Geometry check sheet. Reference: the model listing, model coordinates, mm. A direction names the side the tool comes from. Round coordinates to 2 decimals unless told otherwise and drop trailing zeros. Order: outer loops, then holes, each group sorted by start corner. A loop starts at its lowest first (then second) coordinate and runs counter-clockwise, first axis right, second up.
Autodesk Inventor part; units mm, degrees
ref_plane "YZ Plane" through (0, 0, 0) normal (1, 0, 0) x (0, 1, 0)
ref_plane "XZ Plane" through (0, 0, 0) normal (0, 1, 0) x (-1, 0, 0)
ref_plane "XY Plane" through (0, 0, 0) normal (0, 0, 1) x (1, 0, 0)
sketch "Szkic8" plane through (0, 0, 0) normal (0, 1, 0) x (-1, 0, 0)
  circle A0 centre (0, 0) radius 38.05
  circle A1 centre (0, 0) radius 36.85
  dimension "d53" = 76.1
  dimension "d54" = 1.2
extrude "Wyciągnięcie proste2" add sketch "Szkic8" along normal mid plane 220
sketch "Szkic13" plane through (0, 0, 0) normal (0, 0, 1) x (1, 0, 0)
  circle A0 centre (0, 0) radius 12.5
  circle A1 centre (0, 0) radius 11.3
  dimension "d67" = 25
  dimension "d68" = 1.2
extrude "Wyciągnięcie proste6" add sketch "Szkic13" along normal blind 41
sketch "Szkic14" plane through (0, 0, 41) normal (0, 0, 1) x (1, 0, 0)
  circle A0 centre (0, 0) radius 11.3
extrude "Wyciągnięcie proste7" cut sketch "Szkic14" against normal blind 41
sketch "Szkic15" plane through (0, -110, 0) normal (0, -1, 0) x (1, 0, 0)
  circle A0 centre (0, 0) radius 36.85
extrude "Wyciągnięcie proste8" cut sketch "Szkic15" against normal blind 220
fillet "Zaokrąglenie3" radius 1.2 2 edges at (0, 12.5, 38.05) (0, -12.5, 38.05)
fillet "Zaokrąglenie4" radius 2.4 2 edges at (0.0022, -11.3, 36.85) (0, 11.3, 36.85)
equation "\"d53\" = OD"
equation "\"d54\" = THK"
equation "\"d55\" = L1"
equation "\"d67\" = OD2"
equation "\"d68\" = THK"
equation "\"d69\" = L2"
equation "\"d71\" = L2"
equation "\"d73\" = L1"
equation "\"d75\" = THK"
equation "\"d76\" = 2 * THK"
equation "\"SzerokośćGięciaPodcięcia\" = Grubość"
equation "\"RozmiarPodcięciaNarożnika\" = 4 * Grubość"
equation "\"PromieńPrzejścia\" = PromieńGięcia"
equation "\"Rozmiar_promienia_Jacobiego\" = PromieńGięcia"
equation "\"Wielk_odstępu\" = Grubość"
equation "\"d2\" = PromieńGięcia"
equation "\"d23\" = PromieńGięcia"
equation "\"OD\" = 76.1"
equation "\"THK\" = 1.2"
equation "\"L1\" = 220"
equation "\"L2\" = 41"
equation "\"OD2\" = 25"
properties part number "Trójnik red. krótki  Ø76,1 25 76,1 s=1,2 L=220" material "304"
(1) Draft check along Z on faces 3 (the cylindrical face through (-20.46, -1.54, -32.08)), 4 (the cylindrical face through (7.988, 1.54, -35.974)), 5 (the flat face through (-6, -10, 41)). Enter one of: released by +Z, released by -Z, zero draft, split by the parting line, or undercut.
Returned:
face 3: split by the parting line
face 4: undercut
face 5: released by +Z
(2) Material ranges on line 1 (Z direction, x = 0, y = -20); line 2 (X direction, y = 0, z = 39.65), recorded low to high.
Returned:
line 1: z = -38.05 to -36.85, 36.85 to 38.05
line 2: x = -12.5 to -11.3, 11.3 to 12.5
(3) Sectioned sample at D-D, the plane x = 0. Give the number of separate pieces and of enclosed holes in the cut face, and give its area (3 significant figures).
Returned:
separate pieces: 3
enclosed holes: 0
area: 506 mm2
(4) Sectioned sample at C-C, the plane y = 79.5. Record the cut outline in (x, z), and give its area (3 significant figures).
Returned:
outline: circle Ø76.1 at (0, 0); hole circle Ø73.7 at (0, 0)
area: 282 mm2
(5) Sectioned sample at A-A, the plane z = 0. Record the cut outline in (x, y), and give its area (3 significant figures).
Returned:
outline: (-38.05, -110) - (-36.85, -110) - (-36.85, 110) - (-38.05, 110) - close; (36.85, -110) - (38.05, -110) - (38.05, 110) - (36.85, 110) - close
area: 528 mm2
(6) Set-up check for faces 1 (the cylindrical face through (-2.71, 12.203, 39.329)), 2 (the flat face through (19.9, 110, 31.2)): record each of +Z, -Z, +X, -X, +Y, -Y from which the full face is reachable in a straight line by a thin tool's end or side.
Returned:
face 1: +Z
face 2: +Z, -Z, +X, -X, +Y
(7) Sectioned sample at B-B, the plane x = 29.5. Record the cut outline in (y, z), and give its area (3 significant figures).
Returned:
outline: (-110, -24.03) - (110, -24.03) - (110, -22.08) - (-110, -22.08) - close; (-110, 22.08) - (110, 22.08) - (110, 24.03) - (-110, 24.03) - close
area: 858 mm2
(8) Depth check by flat-ended pin: P1, Ø12, axis at x = -28.5, y = 11, coming from the +Z side; P2, Ø5, axis at y = -57, z = -4, coming from the -X side; P3, Ø20.5, axis at x = 0, y = 0, coming from the -Z side; P4, Ø6, axis at x = 27.5, z = -16.5, coming from the +Y side. Enter the tip coordinate at first touch or a pass-through.
Returned:
P1: stops at z = 30.68
P2: stops at x = -38.02
P3: stops at z = -38.05
P4: passes through
